Here's the drawing with two shaded views (mm, measured from the low corner). I have some questions. A direction names the side the tool comes from. Give positions to 0.01 mm unless a question says otherwise; leave off trailing zeros. Write each loop counter-clockwise with the first axis right and the second up, starting at its lowest first coordinate (ties: lowest second). Pieces come first, ordered by that corner, then holes. Notation, with made-up numbers: (68, 73) - (102, 73) arc R29 ccw to (102, 95) - close; hole circle Ø4 at (-20.75, -15.5). An arc over 180 degrees is marked (long way). Write item = value, one per line.
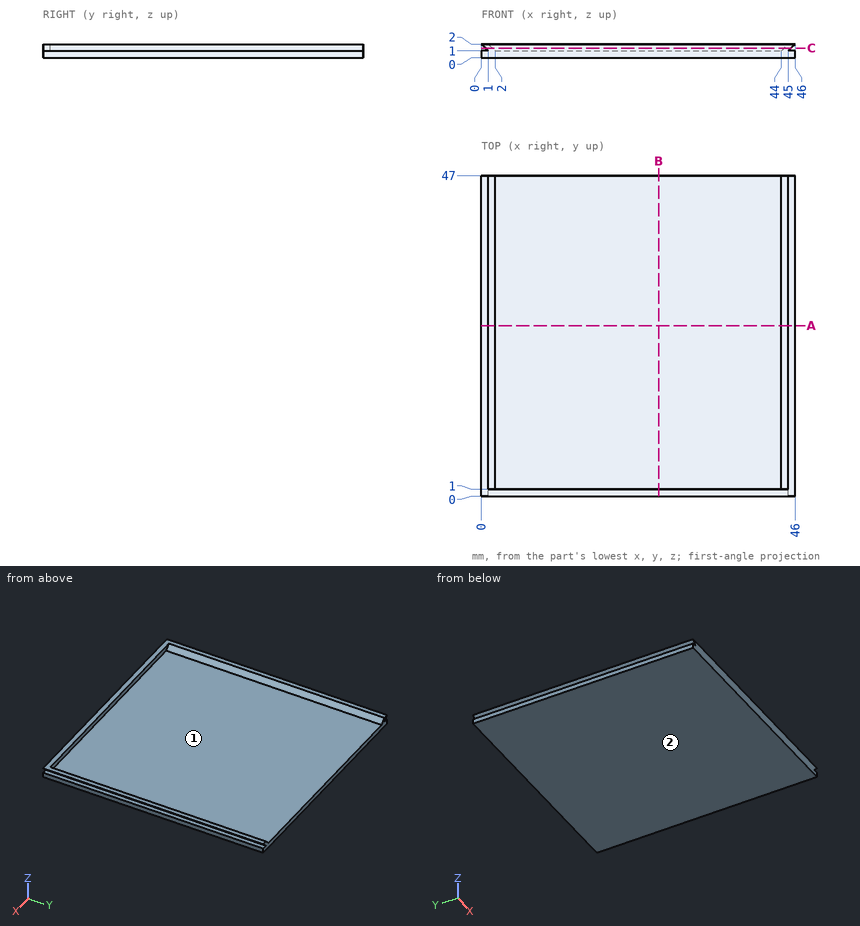
1. If we section it at B-B, the plane x = 26: Please give me the cut outline in (y, z), and give its area (3 significant figures).
Filled sheet:
outline = (0, 0) - (47, 0) - (47, 1) - (1, 1) - (1, 2) - (0, 2) - close
area = 48.0 mm2
2. Which directions (+Z, -Z, +X, -X, +Y, -Y) give clear straight access to the entire face, cutting with the end or side of a thin tool? Please do the marked faces 1 and 2.
Filled sheet:
face_1 = +Z, +Y
face_2 = -Z, +X, -X, +Y, -Y
3. I need wall thicknesses on line 1 (Z direction, x = 41, y = 12.5); line 2 (X direction, y = 35, z = 1.05). Which ranges of each line are inside material? Lowest first, please.
Filled sheet:
line_1 = 0 to 1
line_2 = 0.95 to 1.95, 44.05 to 45.05
4. If we section it at A-A, the plane y = 25: Please give me the cut outline in (x, z).
Filled sheet:
outline = (0, 0) - (46, 0) - (46, 1) - (45, 1) - (46, 2) - (45, 2) - (44, 1) - (2, 1) - (1, 2) - (0, 2) - (1, 1) - (0, 1) - close
5. If we section it at C-C, the plane z = 1.4: Please give me the cut outline in (x, y).
Filled sheet:
outline = (0.6, 0) - (45.4, 0) - (45.4, 47) - (44.4, 47) - (44.4, 1) - (1.6, 1) - (1.6, 47) - (0.6, 47) - close
6. For pin 1 (10 mm diameter, centred on x = 37.5, y = 37.5, fed in from -Z); pin 2 (21 mm diameter, centred on x = 27, y = 33.5, fed in from +Z); pin 3 (0.8 mm diameter, centred on x = 33, z = 1.5, fed in from +Y), each with a flat end and sliding along its axis, tell me the tip position at first contact or that it passes through.
Filled sheet:
pin_1 = 0
pin_2 = 1
pin_3 = 1
